Answer from the drawing. Dimensions are ordinates in mm from the lowest x, y and z of the part. A direction names the side the tool comes from. Round coordinates to 2 decimals unless told otherwise and drop trailing zeros. Loops run counter-clockwise (first coordinate to the right, second up) from the corner with the lowest first, then second, coordinate; pieces in that order, holes last.
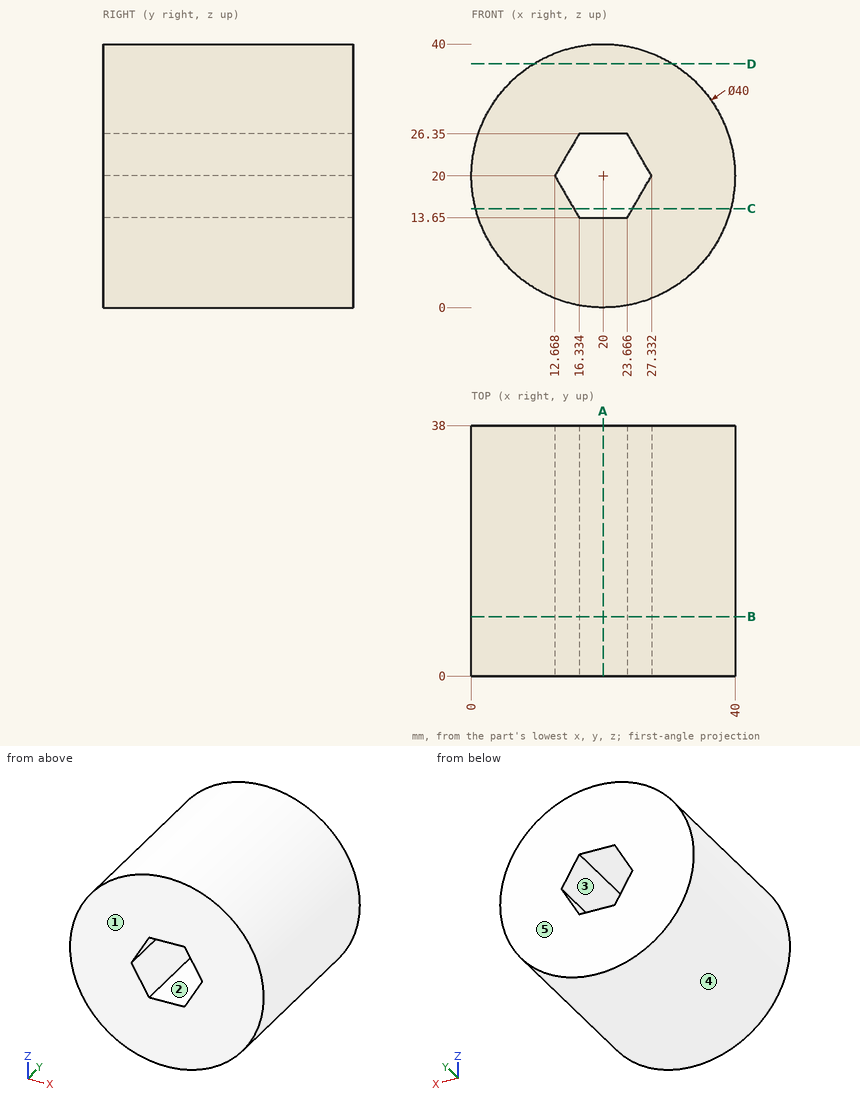
1. Find section A-A (x = 20). Write down the section's boundary in (y, z), then the cut area to 3 significant figures.
Answer key:
outline: (0, 0) - (38, 0) - (38, 13.65) - (0, 13.65) - close; (0, 26.35) - (38, 26.35) - (38, 40) - (0, 40) - close
area: 1,040 mm2
2. Consider probe 1 along X at (y, z) = (35.5, 15.5) (1 decimal); probe 2 along Z at (x, y) = (15.5, 19.5) (1 decimal); probe 3 along X at (y, z) = (23, 23) (1 decimal). Determine where each line is inside the solid, lowest interval first.
Answer key:
probe 1: x = 0.5 to 15.3, 24.7 to 39.5
probe 2: z = 0.5 to 15.1, 24.9 to 39.5
probe 3: x = 0.2 to 14.4, 25.6 to 39.8
3. Find section B-B (y = 9). Write down the section's boundary in (x, z), then the cut area to 3 significant figures.
Answer key:
outline: circle Ø40 at (20, 20); hole (12.67, 20) - (16.33, 13.65) - (23.67, 13.65) - (27.33, 20) - (23.67, 26.35) - (16.33, 26.35) - close
area: 1,120 mm2
4. Find section D-D (z = 37). Write down the section's boundary in (x, y).
Answer key:
outline: (9.46, 0) - (30.54, 0) - (30.54, 38) - (9.46, 38) - close
5. Determine the mould class of the marked faces 3, 4 and 5 for opening direction X: +X half, -X half, draft (parallel to the pull), parting line (faces both ways), or undercut.
Answer key:
face 3: undercut
face 4: parting line
face 5: draft
6. Find section C-C (z = 15). Write down the section's boundary in (x, y) (1 decimal), then the cut area to 3 significant figures.
Answer key:
outline: (0.6, 0) - (15.6, 0) - (15.6, 38) - (0.6, 38) - close; (24.4, 0) - (39.4, 0) - (39.4, 38) - (24.4, 38) - close
area: 1,130 mm2
7. Which of the six approach directions +Z, -Z, +X, -X, +Y, -Y give full straight-line access (tool end or side, diameter ignored) to the marked faces 1 and 2?
Answer key:
face 1: +Z, -Z, +X, -X, -Y
face 2: +Y, -Y
8. Given pin 1 (2 mm diameter, centred on x = 21, y = 25, fed in from -Z); pin 2 (2 mm diameter, centred on x = 21.5, y = 10, fed in from +Z); pin 3 (4 mm diameter, centred on x = 34.5, y = 30.5, fed in from +Z), each flat-ended and moving along its own axis, determine where each tip first touches the part or whether it passes through.
Answer key:
pin 1: stops at z = 0
pin 2: stops at z = 39.99
pin 3: stops at z = 35.61
